```python
from build123d import *

# Parameters (mm, degrees)
F1_DEPTH = 5
F2_R     = 2


with BuildPart() as f1:
    # F0 (on Top) → F1 (new body)
    with BuildSketch(Plane.XY):
        with BuildLine():
            ThreePointArc((3.63717, -5.720129), (5.85243, -3.218601), (6.75, 0))
            ThreePointArc((6.75, 0), (0, 6.761681), (-6.75, 0))
            Line((-6.75, 0), (-6.75, -2.528022))
            Line((-6.75, -2.528022), (-1.75, -2.528022))
            Line((-1.75, -2.528022), (-1.75, 0))
            ThreePointArc((-1.75, 0), (0, 1.75), (1.75, 0))
            ThreePointArc((1.75, 0), (-0.257619, -4.599435), (-3.63717, -8.309419))
            ThreePointArc((-3.63717, -8.309419), (-5.85243, -10.810947), (-6.75, -14.029548))
            ThreePointArc((-6.75, -14.029548), (0, -20.791229), (6.75, -14.029548))
            Line((6.75, -14.029548), (6.75, -11.501526))
            Line((6.75, -11.501526), (1.75, -11.501526))
            Line((1.75, -11.501526), (1.75, -14.029548))
            ThreePointArc((1.75, -14.029548), (0, -15.779548), (-1.75, -14.029548))
            ThreePointArc((-1.75, -14.029548), (0.257619, -9.430112), (3.63717, -5.720129))
        make_face()
    extrude(amount=F1_DEPTH)

    # F2
    f2_edges = [f1.edges().sort_by_distance(p)[0] for p in [
        (-6.75, -2.528022, 2.5),
        (6.75, -11.501526, 2.5),
        (1.75, -11.501526, 2.5),
        (-1.75, -2.528022, 2.5),
    ]]
    fillet(f2_edges, radius=F2_R)


solid = f1.part
```
Could you check a few things on this model? Use its own coordinates, in mm. A direction names the side the tool comes from. Coordinates: 2 decimals unless noted, no trailing zeros. Loops run counter-clockwise (first coordinate to the right, second up) from the corner with the lowest first, then second, coordinate; pieces in that order, holes last. Notation, with made-up numbers: M -9.5,72 L 36.5,72 A22 cw 36.5,104 Z; hole C 71.5,-35 d11. An arc over 180 degrees is marked long. Put each result on its own line as item: value. Start each with the question number.
(1) I need wall thicknesses on line 1 (Y direction, x = -0.5, z = 2.15); line 2 (Y direction, x = 0.5, z = 2.05); line 3 (Y direction, x = 3.25, z = 1.2). Which ranges of each line are inside material? Lowest first, please. Write a range as from..to.
(2) Will these pins go through, and if not, where does the flat tip stop? P1, Ø0.8, axis at x = 4, z = 3, coming from the +Y side; P2, Ø0.5, axis at x = -4.5, z = 1.5, coming from the -Y side; P3, Ø2, axis at x = 2, z = 3.5, coming from the -Y side.
(3) For faces 3 (the face through (-6.18, -1.927, 2.535)), 4 (the face through (6.18, -12.103, 2.535)), 5 (the face through (0.04, -15.78, 2.46)), which set-ups out of +Z, -Z, +X, -X, +Y, -Y let a thin tool reach every point of the face, with its end or its side?
(4) Suppose I cut it at C-C on x = 3. Please give me the cut outline in (y, z).
(5) Suppose I cut it at A-A on x = 1. Please give me the cut outline in (y, z), then the cut area to 3 significant figures.
(6) Thinking about a two-plate mould opening in Y: for faces 1 (the face through (0, -7, 0)), 2 (the face through (-5.83, -10.77, 2.46)), which applies, pulls with the +Y half, pulls with the -Y half, needs draft (parallel to the pull), parting line crosses it, or undercut?
(7) Suppose I cut it at B-B on z = 4.6. Please give me the cut outline in (x, y), then the cut area to 3 significant figures.
(8) Suppose I cut it at D-D on y = -1.75. Please give me the cut outline in (x, z).
Solutions:
1. line 1: y = -20.77..-15.71, -10.73..-4.96, 1.68..6.74
1. line 2: y = -20.77..-15.71, -9.07..-3.3, 1.68..6.74
1. line 3: y = -19.96..-11.57, -6.04..5.93
2. P1: stops at y = 5.72
2. P2: stops at y = -19.29
2. P3: stops at y = -20.72
3. face 3: +Z, -Z, -X
3. face 4: +Z, -Z, +X
3. face 5: +Z, -Z
4. outline: M -20.09,0 L -11.65,0 L -11.65,5 L -20.09,5 Z; M -6.25,0 L 6.06,0 L 6.06,5 L -6.25,5 Z
5. outline: M -20.72,0 L -15.47,0 L -15.47,5 L -20.72,5 Z; M -8.38,0 L -2.23,0 L -2.23,5 L -8.38,5 Z; M 1.44,0 L 6.69,0 L 6.69,5 L 1.44,5 Z
5. area: 83.3 mm2
6. face 1: needs draft
6. face 2: undercut
7. outline: M -6.75,-14.03 A6.75 ccw 6.75,-14.03 L 6.75,-13.5 A2 ccw 4.75,-11.5 L 3.75,-11.5 A2 ccw 1.75,-13.5 L 1.75,-14.03 A1.75 cw -1.75,-14.03 A15.4 cw 3.64,-5.72 A7.44 ccw 6.75,0 A6.75 ccw -6.75,0 L -6.75,-0.53 A2 ccw -4.75,-2.53 L -3.75,-2.53 A2 ccw -1.75,-0.53 L -1.75,0 A1.75 cw 1.75,0 A15.4 cw -3.64,-8.31 A7.44 ccw Z
7. area: 227 mm2
8. outline: M -6.33,0 L -2.17,0 L -2.17,5 L -6.33,5 Z; M 1.19,0 L 6.46,0 L 6.46,5 L 1.19,5 Z
